from build123d import *

# Parameters (mm, degrees)
SKETCH3_W           = 152.4
SKETCH3_H           = 15.875
BOSS_EXTRUDE1_DEPTH = 76.2
SKETCH4_R           = 22.621875
CUT_EXTRUDE1_DEPTH  = 9.525
SKETCH5_R           = 18.0975
CUT_EXTRUDE2_DEPTH  = 109.183203987


with BuildPart() as part:
    # Sketch3 → Boss-Extrude1 (new, symmetric)
    with BuildSketch(Plane.XY):
        Rectangle(SKETCH3_W, SKETCH3_H)
    extrude(amount=BOSS_EXTRUDE1_DEPTH, both=True)

    # Sketch4 → Cut-Extrude1 (cut)
    with BuildSketch(Plane(origin=(0, 7.9375, 0), x_dir=(1, 0, 0), z_dir=(0, 1, 0))):
        with Locations(Location((0, 0, 0), (0, 0, 270))):
            Circle(SKETCH4_R)
    extrude(amount=-CUT_EXTRUDE1_DEPTH, mode=Mode.SUBTRACT)

    # Sketch5 → Cut-Extrude2 (cut, through all)
    with BuildSketch(Plane(origin=(0, -1.5875, 0), x_dir=(1, 0, 0), z_dir=(0, 1, 0))):
        with Locations(Location((0, 0, 0), (0, 0, 270))):
            Circle(SKETCH5_R)
    extrude(amount=-CUT_EXTRUDE2_DEPTH, mode=Mode.SUBTRACT)


solid = part.part
For this review, take the finished solid that the model builds, in its own axes (mm). A direction names the side the tool comes from. Coordinates: 2 decimals unless noted, no trailing zeros. Loops run counter-clockwise (first coordinate to the right, second up) from the corner with the lowest first, then second, coordinate; pieces in that order, holes last. Notation, with made-up numbers: (-39, 62) - (-24, 62) arc R9 cw to (-24, 76) - close; hole circle Ø2 at (63.5, -7). An arc over 180 degrees is marked (long way). Use a Markdown table: item, result. Add a question column.
Item 1: We need section A-A (x = 0). Give the boundary of the cut face in (y, z), and give its area (3 significant figures).
Item 2: Tool access review of faces 1 (the face through (76.2, 0, 1)), 2 (the face through (22.43, 3.24, -2.94)): name each direction out of +Z, -Z, +X, -X, +Y, -Y from which nothing blocks a thin tool from reaching the whole face with its end or side.
Item 3: We need section B-B (z = 0). Give the boundary of the cut face in (x, y).
Item 4: Mouldability with a two-part tool opening along Z and no side actions: class faces 3 (the face through (15.2, -1.588, -10.2)), 4 (the face through (-76.2, 0, 1)), 5 (the face through (17.943, -4.718, -2.356)), 6 (the face through (-1, 0, -76.2)) as pulls with the +Z half, pulls with the -Z half, needs draft (parallel to the pull), parting line crosses it, or undercut.
Item 5: We need section C-C (y = -4). Give the boundary of the cut face in (x, z) (1 decimal).
Item 6: For line 1 (X direction, y = -3.5, z = 0); line 2 (X direction, y = 6, z = 0); line 3 (Z direction, x = -14, y = 3.25), list the stretches that pass through material, from the lowest coordinate up.
Results list:
| question | item | result |
|---|---|---|
| 1 | outline | (-7.94, -76.2) - (7.94, -76.2) - (7.94, -22.62) - (-1.59, -22.62) - (-1.59, -18.1) - (-7.94, -18.1) - close; (-7.94, 18.1) - (-1.59, 18.1) - (-1.59, 22.62) - (7.94, 22.62) - (7.94, 76.2) - (-7.94, 76.2) - close |
| 1 | area | 1,760 mm^2 |
| 2 | face 1 | +Z, -Z, +X, +Y, -Y |
| 2 | face 2 | +Y |
| 3 | outline | (-76.2, -7.94) - (-18.1, -7.94) - (-18.1, -1.59) - (-22.62, -1.59) - (-22.62, 7.94) - (-76.2, 7.94) - close; (18.1, -7.94) - (76.2, -7.94) - (76.2, 7.94) - (22.62, 7.94) - (22.62, -1.59) - (18.1, -1.59) - close |
| 4 | face 3 | undercut |
| 4 | face 4 | needs draft |
| 4 | face 5 | undercut |
| 4 | face 6 | pulls with the -Z half |
| 5 | outline | (-76.2, -76.2) - (76.2, -76.2) - (76.2, 76.2) - (-76.2, 76.2) - close; hole circle Ø36.2 at (0, 0) |
| 6 | line 1 | x = -76.2 to -18.1, 18.1 to 76.2 |
| 6 | line 2 | x = -76.2 to -22.62, 22.62 to 76.2 |
| 6 | line 3 | z = -76.2 to -17.77, 17.77 to 76.2 |
